```python
from build123d import *

# Parameters (mm, degrees)
SKETCH4_R           = 10
BOSS_EXTRUDE1_DEPTH = 20
SKETCH5_R           = 10
BOSS_EXTRUDE2_DEPTH = 15


with BuildPart() as part:
    # Sketch4 → Boss-Extrude1 (new body)
    with BuildSketch(Plane(origin=(0, 0, 0), x_dir=(1, 0, 0), z_dir=(0, 1, 0))):
        with BuildLine():
            Line((-77.28011811, -56.673598022), (-77.28011811, 23.326401978))
            Line((-77.28011811, 23.326401978), (-16.966387776, 23.326401978))
            ThreePointArc((-16.966387776, 23.326401978), (-3.737631221, 28.326401978), (2.876747057, 40.826401978))
            ThreePointArc((2.876747057, 40.826401978), (12.736944948, 55.656750215), (30.512681706, 56.745747))
            Line((30.512681706, 56.745747), (160.512681706, 1.745747))
            ThreePointArc((160.512681706, 1.745747), (172.71988189, -16.673598022), (160.512681706, -35.092943043))
            Line((160.512681706, -35.092943043), (30.512681706, -90.092943043))
            ThreePointArc((30.512681706, -90.092943043), (12.736944948, -89.003946259), (2.876747057, -74.173598022))
            ThreePointArc((2.876747057, -74.173598022), (-3.737631221, -61.673598022), (-16.966387776, -56.673598022))
            Line((-16.966387776, -56.673598022), (-77.28011811, -56.673598022))
        make_face()
        with Locations(Location((-57.28011811, -16.673598022, 0), (0, 0, 270))):
            Circle(SKETCH4_R, mode=Mode.SUBTRACT)
    extrude(amount=BOSS_EXTRUDE1_DEPTH)

    # Sketch5 → Boss-Extrude2 (add)
    with BuildSketch(Plane.XY.offset(56.673598022)):
        with BuildLine():
            Line((-77.28011811, 20), (-77.28011811, 60))
            ThreePointArc((-77.28011811, 60), (-60.595178298, 79.723345962), (-38.379080515, 66.538407896))
            Line((-38.379080515, 66.538407896), (-22.28011811, 20))
            Line((-22.28011811, 20), (-77.28011811, 20))
        make_face()
        with Locations((-57.28011811, 60)):
            Circle(SKETCH5_R, mode=Mode.SUBTRACT)
    extrude(amount=-BOSS_EXTRUDE2_DEPTH)


solid = part.part
```
Input: part model. Units: mm. Frame: model coordinates. A direction names the side the tool comes from. Give positions to 0.01 mm unless a question says otherwise; leave off trailing zeros. Loops run counter-clockwise (first coordinate to the right, second up) from the corner with the lowest first, then second, coordinate; pieces in that order, holes last. Notation, with made-up numbers: (-13, 41.5) -> (-6, 41.5) arc R19 ccw to (-6, 57.5) -> close; hole circle Ø11 at (-34, -8). An arc over 180 degrees is marked (long way). Use a Markdown table: item, result.
Q1. Section query C-C, the plane y = 17.5. Return the cut outline in (x, z), plus the area to 3 significant figures.
Entries:
| item | result |
|---|---|
| outline | (-77.28, -23.33) -> (-16.97, -23.33) arc R20 cw to (2.88, -40.83) arc R20 ccw to (30.51, -56.75) -> (160.51, -1.75) arc R20 ccw to (160.51, 35.09) -> (30.51, 90.09) arc R20 ccw to (2.88, 74.17) arc R20 cw to (-16.97, 56.67) -> (-77.28, 56.67) -> close; hole circle Ø20 at (-57.28, 16.67) |
| area | 22,500 mm² |
Q2. Section query D-D, the plane x = 80.5. Return the cut outline in (y, z).
Entries:
| item | result |
|---|---|
| outline | (0, -35.6) -> (20, -35.6) -> (20, 68.94) -> (0, 68.94) -> close |
Q3. First-contact query: P1, Ø8, axis at x = 44, z = 33.5, coming from the +Y side; P2, Ø18, axis at x = -57.28, y = 60, coming from the -Z side; P3, Ø8, axis at x = 57, y = 11, coming from the -Z side; P4, Ø3, axis at y = 10.5, z = -31.5, coming from the -X side. Flat tips, straight axial feed; report the tip coordinate or a pass-through.
Entries:
| item | result |
|---|---|
| P1 | stops at y = 20 |
| P2 | passes through |
| P3 | stops at z = -47.23 |
| P4 | stops at x = -2.05 |
Q4. Ray query, probe 1 along Y at (x, z) = (117, 3); probe 2 along Z at (x, y) = (-47, 6); probe 3 along Z at (x, y) = (-0.5, 7). Return the intervals inside material, ascending. Write a range as from..to.
Entries:
| item | result |
|---|---|
| probe 1 | y = 0..20 |
| probe 2 | z = -23.33..56.67 |
| probe 3 | z = -31.97..65.32 |
Q5. Section query B-B, the plane y = 56. Return the cut outline in (x, z), plus the area to 3 significant figures.
Entries:
| item | result |
|---|---|
| outline | (-77.28, 41.67) -> (-66.45, 41.67) -> (-66.45, 56.67) -> (-77.28, 56.67) -> close; (-48.11, 41.67) -> (-34.73, 41.67) -> (-34.73, 56.67) -> (-48.11, 56.67) -> close |
| area | 363 mm² |
Q6. Access query for faces 5 (the flat face through (-53, 32, 56.674)), 6 (the cylindrical face through (-65.22, 53.92, 49.28)), 7 (the flat face through (-48, 10, -23.326)). Directions: +Z, -Z, +X, -X, +Y, -Y. A direction counts if a zero-diameter tool reaches every point of the face in a straight line with its end or side. Return the directions, or none.
Entries:
| item | result |
|---|---|
| face 5 | +Z, -X, +Y, -Y |
| face 6 | +Z, -Z |
| face 7 | -Z, -X, +Y, -Y |
Q7. Section query A-A, the plane z = 9.5. Return the cut outline in (x, y), plus the area to 3 significant figures.
Entries:
| item | result |
|---|---|
| outline | (-77.28, 0) -> (-64.25, 0) -> (-64.25, 20) -> (-77.28, 20) -> close; (-50.31, 0) -> (171.39, 0) -> (171.39, 20) -> (-50.31, 20) -> close |
| area | 4,690 mm² |
Q8. Pull-direction query (Z, two-part tool) for faces 1 (the cylindrical face through (-47.365, 9.86, 15.372)), 2 (the flat face through (-56, 44, 41.674)), 3 (the flat face through (-30.44, 43.59, 49.28)), 4 (the flat face through (96.42, 9.86, 62.21)); classes: pulls with the +Z half, pulls with the -Z half, needs draft (parallel to the pull), parting line crosses it, or undercut.
Entries:
| item | result |
|---|---|
| face 1 | undercut |
| face 2 | pulls with the -Z half |
| face 3 | needs draft |
| face 4 | pulls with the +Z half |
